The listing builds one solid part. Answer for the finished solid, in the listing's coordinates (mm). A direction names the side the tool comes from. Coordinates: 2 decimals unless noted, no trailing zeros. Order: outer loops, then holes, each group sorted by start corner. A loop starts at its lowest first (then second) coordinate and runs counter-clockwise, first axis right, second up.
```python
from build123d import *

# Parameters (mm, degrees)
F1_DEPTH  = 3.048
F2_SIZE   = 1.778
F3_W      = 7.570412
F3_H      = 3.080346
F4_DEPTH  = 0.508
F4_FACE_W = 7.570412
F4_FACE_H = 3.080346
F5_DEPTH  = 2.032


with BuildPart() as f1:
    # F0 (on Top) → F1 (new body)
    with BuildSketch(Plane.XY):
        Polygon((-18.5674, 0), (0, 0), (18.563472, 0), (0, 28.34343), align=None)
    extrude(amount=F1_DEPTH)

    # F2
    f2_edges = [f1.edges().sort_by_distance(p)[0] for p in [
        (-9.2837, 14.171715, 3.048),
        (-0.001964, 0, 3.048),
        (9.281736, 14.171715, 3.048),
    ]]
    chamfer(f2_edges, length=F2_SIZE)

    # F3 (on face) → F4 (cut)
    with BuildSketch(Plane.XY.offset(3.048)):
        with Locations((0, 9.814435)):
            Rectangle(F3_W, F3_H)
    extrude(amount=-F4_DEPTH, mode=Mode.SUBTRACT)

    # F4_face (on face) → F5 (cut)
    with BuildSketch(Plane(origin=(0, 9.814435, 2.54), x_dir=(1, 0, 0), z_dir=(0, 0, 1))):
        Rectangle(F4_FACE_W, F4_FACE_H)
    extrude(amount=-F5_DEPTH, mode=Mode.SUBTRACT)


solid = f1.part
```
1) Straight lines are drawn through the part: probe 1 along Z at (x, y) = (2, 10.25); probe 2 along Y at (x, z) = (3.5, 1.95); probe 3 along X at (y, z) = (12.75, 0.35). For each, find the intervals that lie inside material, in ascending order.
2) A cutting plane is placed at A-A, the plane z = 2. Write down the section's boundary in (x, y), plus the area to 3 significant figures.
3) For faces 5 (the flat face through (0, 14, 3.048)), 6 (the flat face through (3.785, 10, 2)), determine the directions among +Z, -Z, +X, -X, +Y, -Y from which every point of the face is accessible in a straight line to the end or side of a thin tool.
4) A cutting plane is placed at B-B, the plane y = 17.25. Write down the section's boundary in (x, z).
5) Each of these flat-tipped pins is pushed along its axis until it touches: P1, Ø4, axis at x = 9.5, y = 16.5, coming from the -Z side; P2, Ø0.9, axis at x = -1, y = 10, coming from the +Z side; P3, Ø1, axis at y = 5, z = 1.5, coming from the +X side; P4, Ø0.8, axis at y = 10.5, z = 1.5, coming from the -X side. Where does it stop, or does it pass through?
6) A cutting plane is placed at C-C, the plane x = 2. Write down the section's boundary in (y, z), plus the area to 3 significant figures.
7) A cutting plane is placed at D-D, the plane x = -2. Write down the section's boundary in (y, z).
8) The mould has two halves that part along X. Classify faces 1 (the flat face through (0, 0, 1)), 2 (the flat face through (-8.4, 13.88, 2.17)), 3 (the flat face through (-3.785, 10, 2)), 4 (the flat face through (0, 10, 0.508)): released by +X, released by -X, zero draft, split by the parting line, or undercut.
Working result:
1. probe 1: z = 0 to 0.51
1. probe 2: y = 0.68 to 8.27, 11.35 to 21.76
1. probe 3: x = -10.22 to 10.21
2. outline: (-17.22, 0.73) - (17.21, 0.73) - (0, 27.01) - close; hole (-3.79, 8.27) - (3.79, 8.27) - (3.79, 11.35) - (-3.79, 11.35) - close
2. area: 429 mm2
3. face 5: +Z, +X, -X, +Y, -Y
3. face 6: +Z
4. outline: (-7.27, 0) - (7.27, 0) - (7.27, 1.27) - (5.14, 3.05) - (-5.14, 3.05) - (-7.27, 1.27) - close
5. P1: stops at z = 0
5. P2: stops at z = 0.51
5. P3: stops at x = 15.58
5. P4: stops at x = -11.9
6. outline: (0, 0) - (25.29, 0) - (25.29, 1.27) - (22.04, 3.05) - (11.35, 3.05) - (11.35, 0.51) - (8.27, 0.51) - (8.27, 3.05) - (1.78, 3.05) - (0, 1.27) - close
6. area: 64.8 mm2
7. outline: (0, 0) - (25.29, 0) - (25.29, 1.27) - (22.05, 3.05) - (11.35, 3.05) - (11.35, 0.51) - (8.27, 0.51) - (8.27, 3.05) - (1.78, 3.05) - (0, 1.27) - close
8. face 1: zero draft
8. face 2: released by -X
8. face 3: undercut
8. face 4: undercut
